Design review of the part built by this model. Coordinates are the model's own, in mm. Face numbers are marked on the shaded views. A direction names the side the tool comes from. Coordinates: 2 decimals unless noted, no trailing zeros. Order: outer loops, then holes, each group sorted by start corner. A loop starts at its lowest first (then second) coordinate and runs counter-clockwise, first axis right, second up. Notation, with made-up numbers: M 0,77.25 L 46,77.25 A26 ccw 46,101.25 Z; hole C -26,77 d1. An arc over 180 degrees is marked long. Answer in a Markdown table with one row per item.
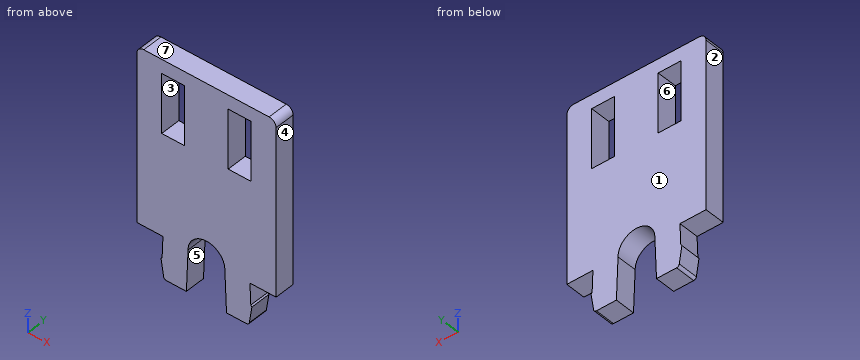
from build123d import *

# Parameters (mm, degrees)
F0_W     = 3.3
F0_H     = 8.5
F1_DEPTH = 2.9


with BuildPart() as f1:
    # F0 (on Front) → F1 (new body)
    with BuildSketch(Plane.XZ):
        with BuildLine():
            Line((-10, 24), (-10, 0))
            Line((-10, 0), (-6.246776, 0))
            Line((-6.246776, 0), (-6.367, -3.05))
            Line((-6.367, -3.05), (-6.525, -3.25))
            Line((-6.525, -3.25), (-6.152377, -5.661093))
            ThreePointArc((-6.152377, -5.661093), (-6.017418, -5.903675), (-5.75707, -6))
            Line((-5.75707, -6), (-2.880486, -6))
            Line((-2.880486, -6), (-2.643981, 0))
            ThreePointArc((-2.643981, 0), (0, 2.643981), (2.643981, 0))
            Line((2.643981, 0), (2.880486, -6))
            Line((2.880486, -6), (5.75707, -6))
            ThreePointArc((5.75707, -6), (6.017418, -5.903675), (6.152377, -5.661093))
            Line((6.152377, -5.661093), (6.525, -3.25))
            Line((6.525, -3.25), (6.367, -3.05))
            Line((6.367, -3.05), (6.246776, 0))
            Line((6.246776, 0), (10, 0))
            Line((10, 0), (10, 24))
            ThreePointArc((10, 24), (9.707107, 24.707107), (9, 25))
            Line((9, 25), (-9, 25))
            ThreePointArc((-9, 25), (-9.707107, 24.707107), (-10, 24))
        make_face()
        with Locations((-4.775, 18.75)):
            Rectangle(F0_W, F0_H, mode=Mode.SUBTRACT)
        with Locations((4.775, 18.75)):
            Rectangle(F0_W, F0_H, mode=Mode.SUBTRACT)
    extrude(amount=F1_DEPTH)


solid = f1.part
(1) Add section C-C, the plane y = -1.6. Give the boundary of the cut face in (x, z) (3 decimals), and give its area (3 significant figures).
Return value:
| item | result |
|---|---|
| outline | M -10,0 L -6.247,0 L -6.367,-3.05 L -6.525,-3.25 L -6.152,-5.661 A0.4 ccw -5.757,-6 L -2.88,-6 L -2.644,0 A2.644 cw 2.644,0 L 2.88,-6 L 5.757,-6 A0.4 ccw 6.152,-5.661 L 6.525,-3.25 L 6.367,-3.05 L 6.247,0 L 10,0 L 10,24 A1 ccw 9,25 L -9,25 A1 ccw -10,24 Z; hole M -6.425,14.5 L -3.125,14.5 L -3.125,23 L -6.425,23 Z; hole M 3.125,14.5 L 6.425,14.5 L 6.425,23 L 3.125,23 Z |
| area | 475 mm2 |
(2) Add section A-A, the plane z = 18. Give the boundary of the cut face in (x, y) (3 decimals), and give its area (3 significant figures).
Return value:
| item | result |
|---|---|
| outline | M -10,-2.9 L -6.425,-2.9 L -6.425,0 L -10,0 Z; M -3.125,-2.9 L 3.125,-2.9 L 3.125,0 L -3.125,0 Z; M 6.425,-2.9 L 10,-2.9 L 10,0 L 6.425,0 Z |
| area | 38.9 mm2 |
(3) Draft analysis for pull direction X (two halves, no side actions). For the marked faces 1, 2, 3 and 4, state which applies: pulls with the +X half, pulls with the -X half, needs draft (parallel to the pull), parting line crosses it, or undercut.
Return value:
| item | result |
|---|---|
| face 1 | needs draft |
| face 2 | pulls with the -X half |
| face 3 | undercut |
| face 4 | pulls with the +X half |
(4) Add section B-B, the plane x = 4.25. Give the boundary of the cut face in (y, z).
Return value:
| item | result |
|---|---|
| outline | M -2.9,-6 L 0,-6 L 0,14.5 L -2.9,14.5 Z; M -2.9,23 L 0,23 L 0,25 L -2.9,25 Z |
(5) Insertion check: pin 1 Ø1.4 at (x, y) = (7.5, -1) entering from -Z. The pin has a flat end and moves straight along its axis. Give the tip position at first contact, or say it passes through.
Return value:
| item | result |
|---|---|
| pin 1 | stops at z = 0 |
(6) For line 1 along X through (y, z) = (-0.65, 18.5) (3 decimals); line 2 along Z through (x, y) = (4.25, -1.4); line 3 along Z through (x, y) = (7.5, -0.3), list the stretches that pass through material, from the lowest coordinate up. Write a range as from..to.
Return value:
| item | result |
|---|---|
| line 1 | x = -10..-6.425, -3.125..3.125, 6.425..10 |
| line 2 | z = -6..14.5, 23..25 |
| line 3 | z = 0..25 |
(7) Add section D-D, the plane z = 1. Give the boundary of the cut face in (x, y).
Return value:
| item | result |
|---|---|
| outline | M -10,-2.9 L -2.45,-2.9 L -2.45,0 L -10,0 Z; M 2.45,-2.9 L 10,-2.9 L 10,0 L 2.45,0 Z |
(8) For the marked faces 5, 6 and 7, list the 3-axis set-ups (+Z, -Z, +X, -X, +Y, -Y) from which the entire face can be reached by the end or side of a thin tool; tool diameter is ignored.
Return value:
| item | result |
|---|---|
| face 5 | -Z, +Y, -Y |
| face 6 | +Y, -Y |
| face 7 | +Z, +X, -X, +Y, -Y |
